Autodesk Inventor part; units mm, degrees
ref_plane "YZ Plane" through (0, 0, 0) normal (1, 0, 0) x (0, 1, 0)
ref_plane "XZ Plane" through (0, 0, 0) normal (0, 1, 0) x (-1, 0, 0)
ref_plane "XY Plane" through (0, 0, 0) normal (0, 0, 1) x (1, 0, 0)
sketch "Sketch1" plane through (0, 0, 0) normal (1, 0, 0) x (0, 1, 0)
  circle A0 centre (0, 0) radius 4
  dimension "d0" = 8
extrude "Extrusion1" add sketch "Sketch1" along normal blind 9.8
sketch "Sketch2" plane through (9.8, 0, 0) normal (1, 0, 0) x (0, 0, -1)
  circle A0 centre (0, 0) radius 10
  circle A1 centre (0, 0) radius 6.5 construction
  circle A2 centre (0, 6.5) radius 1.5
  circle A3 centre (-5.6292, -3.25) radius 1.5
  circle A4 centre (5.6292, -3.25) radius 1.5
  dimension "d4" = 13
  dimension "d3" = 20
  dimension "d5" = 3
  dimension "d8" = 360
extrude "Extrusion2" add sketch "Sketch2" against normal blind 3.2
sketch "Sketch3" plane through (9.8, 0, 0) normal (1, 0, 0) x (0, 0, -1)
  circle A0 centre (0, 0) radius 2.5
  dimension "d12" = 5
extrude "Extrusion3" cut sketch "Sketch3" against normal through all
sketch "Sketch4" plane through (9.8, 0, 0) normal (1, 0, 0) x (0, 0, -1)
  line L0 (8.1454, -10.691) -> (-8.1454, -10.691)
  line L1 (-8.1454, -10.691) -> (-8.1454, -9.309)
  line L2 (-8.1454, -9.309) -> (8.1454, -9.309)
  line L3 (8.1454, -9.309) -> (8.1454, -10.691)
  circle A0 centre (0, 0) radius 10
  line L4 (8.1454, -10.691) -> (-8.1454, -9.309) construction
  line L5 (-8.1454, -10.691) -> (8.1454, -9.309) construction
  point P0 (0, -10)
extrude "Extrusion4" cut sketch "Sketch4" against normal through all contours L0 L1 L2 A0 L3 | A0 L2 picked at (-0.4144, -9.5135)
properties part number "Nut"
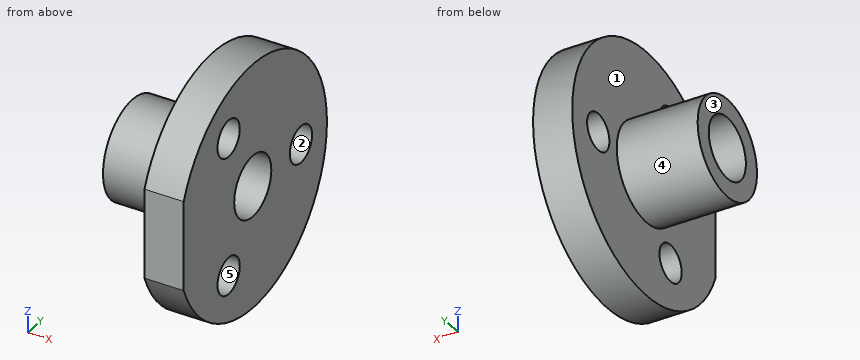
CAD build for the part. Positions are in the model's coordinates, mm. Face numbers are marked on the shaded views. A direction names the side the tool comes from. Round coordinates to 2 decimals unless told otherwise and drop trailing zeros. Order: outer loops, then holes, each group sorted by start corner. A loop starts at its lowest first (then second) coordinate and runs counter-clockwise, first axis right, second up. Notation, with made-up numbers: (23, 10) - (34, 10) arc R27 cw to (34, 49) - close; hole circle Ø2 at (24.5, 31.5). An arc over 180 degrees is marked (long way). Answer in a Markdown table with one row per item. Add a question column.
(1) Band-saw the part on D-D on x = 1.5. List the corners of the cut face in (y, z).
(2) Band-saw the part on C-C on x = 8.5. List the corners of the cut face in (y, z), and give its area (3 significant figures).
(3) Band-saw the part on B-B on z = 0. List the corners of the cut face in (x, y), and give its area (3 significant figures).
(4) Probe L1, parallel to Y at x = 8.55, z = 0; L2, parallel to Y at x = 2.25, z = 0; L3, parallel to X at y = 0.5, z = 7.5. List the from-to ranges inside material, lowest first. Write a range as [from, to].
(5) Mould opens along Z. For the marked faces 3, 4 and 5 say: +Z half, -Z half, draft (parallel to the pull), parting line (faces both ways), or undercut.
(6) Band-saw the part on A-A on y = 0. List the corners of the cut face in (x, z).
(7) Drop flat-ended pins along their axis: pin 1 Ø3 at (x, z) = (7.5, 6.5) entering from +Y; pin 2 Ø3.5 at (y, z) = (-3.25, -5.63) entering from -X; pin 3 Ø4 at (x, y) = (7, 6) entering from +Z; pin 4 Ø3 at (y, z) = (0, 0) entering from +X. Give the stop position or say it passes through.
(8) 3-axis set-ups, long thin cutter, end or side, ignore diameter. For the marked faces 1 and 2: which of +Z, -Z, +X, -X, +Y, -Y reach the whole face in a straight line?
Data:
| question | item | result |
|---|---|---|
| 1 | outline | circle Ø8 at (0, 0); hole circle Ø5 at (0, 0) |
| 2 | outline | (-9.31, -3.65) arc R10 ccw (long way) to (-9.31, 3.65) - close; hole circle Ø3 at (-3.25, -5.63); hole circle Ø3 at (-3.25, 5.63); hole circle Ø5 at (0, 0); hole circle Ø3 at (6.5, 0) |
| 2 | area | 270 mm^2 |
| 3 | outline | (0, -4) - (6.6, -4) - (6.6, -9.31) - (9.8, -9.31) - (9.8, -2.5) - (0, -2.5) - close; (0, 2.5) - (9.8, 2.5) - (9.8, 5) - (6.6, 5) - (6.6, 4) - (0, 4) - close; (6.6, 8) - (9.8, 8) - (9.8, 10) - (6.6, 10) - close |
| 3 | area | 56.0 mm^2 |
| 4 | L1 | y = [-9.31, -2.5], [2.5, 5], [8, 10] |
| 4 | L2 | y = [-4, -2.5], [2.5, 4] |
| 4 | L3 | x = [6.6, 9.8] |
| 5 | face 3 | draft |
| 5 | face 4 | parting line |
| 5 | face 5 | undercut |
| 6 | outline | (0, -4) - (6.6, -4) - (6.6, -10) - (9.8, -10) - (9.8, -2.5) - (0, -2.5) - close; (0, 2.5) - (9.8, 2.5) - (9.8, 10) - (6.6, 10) - (6.6, 4) - (0, 4) - close |
| 7 | pin 1 | stops at y = 8.66 |
| 7 | pin 2 | stops at x = 6.6 |
| 7 | pin 3 | stops at z = 9.17 |
| 7 | pin 4 | passes through |
| 8 | face 1 | -X |
| 8 | face 2 | +X, -X |
